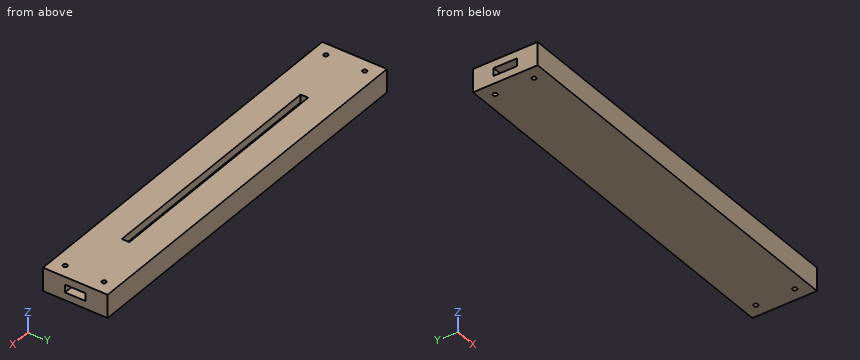
from build123d import *

# Parameters (mm, degrees)
SKETCH_W              = 150
SKETCH_H              = 25
PAD_DEPTH             = 3
PAD001_DEPTH          = 3
SKETCH004_W           = 150
SKETCH004_H           = 25
SKETCH004_W_2         = 96
SKETCH004_H_2         = 2.9
PAD002_DEPTH          = 3
SKETCH005_R           = 0.85
POCKET_DEPTH          = 313.671314
POLARPATTERN_COUNT    = 2
POLARPATTERN001_COUNT = 2
POLARPATTERN002_COUNT = 2


with BuildPart() as part:
    # Sketch → Pad (new body)
    with BuildSketch(Plane.XY):
        Rectangle(SKETCH_W, SKETCH_H)
    extrude(amount=PAD_DEPTH)

    # Sketch001 (on Face6 of Pad) → Pad001 (join)
    with BuildSketch(Plane.XY.offset(3)):
        Polygon((-75, 12.5), (75, 12.5), (75, 4), (50, 4), (50, 5), (-50, 5), (-50, 4), (-52.25, 4), (-52.25, 9.2), (-72.25, 9.2), (-72.25, 4.5), (-75, 4.5), align=None)
        Polygon((-75, -12.5), (75, -12.5), (75, -4), (50, -4), (50, -5), (-50, -5), (-50, -4), (-52.25, -4), (-52.25, -9.2), (-72.25, -9.2), (-72.25, -4.5), (-75, -4.5), align=None)
    extrude(amount=PAD001_DEPTH)

    # Sketch004 (on Face12 of Pad001) → Pad002 (join)
    with BuildSketch(Plane.XY.offset(6)):
        Rectangle(SKETCH004_W, SKETCH004_H)
        Rectangle(SKETCH004_W_2, SKETCH004_H_2, mode=Mode.SUBTRACT)
    extrude(amount=PAD002_DEPTH)

    # Sketch005 (on Face34 of Pad002) → Pocket (cut, through all)
    with BuildSketch(Plane.XY.offset(9)):
        with Locations((-70, 7.5)):
            Circle(SKETCH005_R)
    pocket = extrude(amount=-POCKET_DEPTH, mode=Mode.SUBTRACT)

    # PolarPattern: Pocket ×2 about axis
    polarpattern_axis = Axis((0, 0, 9), (0, 0, 1))
    for i in range(1, POLARPATTERN_COUNT):
        add(pocket.rotate(polarpattern_axis, i * 360 / POLARPATTERN_COUNT), mode=Mode.SUBTRACT)

    # PolarPattern001: Pocket ×2 about axis
    polarpattern001_axis = Axis((0, 0, 0), (0, 1, 0))
    for i in range(1, POLARPATTERN001_COUNT):
        add(pocket.rotate(polarpattern001_axis, i * 360 / POLARPATTERN001_COUNT), mode=Mode.SUBTRACT)

    # PolarPattern002: Pocket ×2 about axis
    polarpattern002_axis = Axis((0, 0, 0), (1, 0, 0))
    for i in range(1, POLARPATTERN002_COUNT):
        add(pocket.rotate(polarpattern002_axis, i * 360 / POLARPATTERN002_COUNT), mode=Mode.SUBTRACT)


solid = part.part
Here's how the part is built. I have some questions about the finished solid (model axes, mm). Round coordinates to 2 decimals unless told otherwise and drop trailing zeros. Loops run counter-clockwise (first coordinate to the right, second up) from the corner with the lowest first, then second, coordinate; pieces in that order, holes last. Notation, with made-up numbers: (60.25, 62.5) - (78.25, 62.5) arc R11 ccw to (78.25, 74.5) - close; hole circle Ø2 at (84.5, 25). An arc over 180 degrees is marked (long way). One line per question, with ' | ' between items. Start each with the question number.
Q1. I want a section at B-B (x = -14). Write out the boundary of the cut face in (y, z).
Q2. Please list where these lines run through material, in increasing order: line 1 (X direction, y = -7.5, z = 4.25); line 2 (X direction, y = -7.5, z = 1.05); line 3 (Y direction, x = -70, z = 6.9). Write a range as [from, to].
Q3. Will these pins go through, and if not, where does the flat tip stop? pin 1 (2 mm diameter, centred on x = -70, y = 7.5, fed in from +Z); pin 2 (1.4 mm diameter, centred on x = -70, y = 7.5, fed in from -Z).
Q4. I want a section at A-A (x = 52.5). Write out the boundary of the cut face in (y, z), then the cut area to 3 significant figures.
Response values:
1) outline: (-12.5, 0) - (12.5, 0) - (12.5, 9) - (1.45, 9) - (1.45, 6) - (5, 6) - (5, 3) - (-5, 3) - (-5, 6) - (-1.45, 6) - (-1.45, 9) - (-12.5, 9) - close
2) line 1: x = [-75, -72.25], [-52.25, 69.15], [70.85, 75] | line 2: x = [-75, -70.85], [-69.15, 69.15], [70.85, 75] | line 3: y = [-12.5, -8.35], [-6.65, 6.65], [8.35, 12.5]
3) pin 1: stops at z = 9 | pin 2: passes through
4) outline: (-12.5, 0) - (12.5, 0) - (12.5, 9) - (-12.5, 9) - close; hole (-4, 3) - (4, 3) - (4, 6) - (-4, 6) - close | area: 201 mm²
